```python
from build123d import *

# Parameters (mm, degrees)
SKETCH1_W           = 120
SKETCH1_H           = 70
BOSS_EXTRUDE1_DEPTH = 2
SKETCH3_R           = 3.5
CUT_EXTRUDE1_DEPTH  = 3
SKETCH6_R           = 2
BOSS_EXTRUDE2_DEPTH = 11
SKETCH4_R           = 3.25
CUT_EXTRUDE2_DEPTH  = 11


with BuildPart() as part:
    # Sketch1 → Boss-Extrude1 (new body)
    with BuildSketch(Plane(origin=(0, 0, 0), x_dir=(1, 0, 0), z_dir=(0, 1, 0))):
        Rectangle(SKETCH1_W, SKETCH1_H)
    extrude(amount=BOSS_EXTRUDE1_DEPTH)

    # Sketch3 → Cut-Extrude1 (cut)
    with BuildSketch(Plane(origin=(0, 2, 0), x_dir=(1, 0, 0), z_dir=(0, 1, 0))):
        with Locations(Location((-53.5, 28.5, 0), (0, 0, 270))):
            Circle(SKETCH3_R)
        with Locations(Location((53.5, 28.5, 0), (0, 0, 270))):
            Circle(SKETCH3_R)
        with Locations(Location((-53.5, -28.5, 0), (0, 0, 270))):
            Circle(SKETCH3_R)
        with Locations(Location((53.5, -28.5, 0), (0, 0, 270))):
            Circle(SKETCH3_R)
    extrude(amount=-CUT_EXTRUDE1_DEPTH, mode=Mode.SUBTRACT)

    # Sketch6 → Boss-Extrude2 (add)
    with BuildSketch(Plane(origin=(0, 2, 0), x_dir=(1, 0, 0), z_dir=(0, 1, 0))):
        with Locations(Location((0, -13, 0), (0, 0, 270))):
            Circle(SKETCH6_R)
        with Locations(Location((0, 13, 0), (0, 0, 270))):
            Circle(SKETCH6_R)
    extrude(amount=-BOSS_EXTRUDE2_DEPTH)

    # Sketch4 → Cut-Extrude2 (cut)
    with BuildSketch(Plane(origin=(0, 2, 0), x_dir=(1, 0, 0), z_dir=(0, 1, 0))):
        with Locations(Location((-27.054448087, -13.122273409, 0), (0, 0, 270))):
            Circle(SKETCH4_R)
        with Locations(Location((-27.023483048, -0.10764713, 0), (0, 0, 270))):
            Circle(SKETCH4_R)
        with Locations(Location((-27.081562274, 12.864019897, 0), (0, 0, 270))):
            Circle(SKETCH4_R)
        with Locations(Location((-13.567081484, 0, 0), (0, 0, 270))):
            Circle(SKETCH4_R)
        with Locations(Location((-13.567081484, -13, 0), (0, 0, 270))):
            Circle(SKETCH4_R)
        with Locations(Location((-13.567081484, 13, 0), (0, 0, 270))):
            Circle(SKETCH4_R)
        with Locations(Location((0, 0, 0), (0, 0, 270))):
            Circle(SKETCH4_R)
    extrude(amount=-CUT_EXTRUDE2_DEPTH, mode=Mode.SUBTRACT)


solid = part.part
```
Geometry: final body of the model. Coordinates: model frame, mm. A direction names the side the tool comes from. Coordinates: 2 decimals unless noted, no trailing zeros. Order: outer loops, then holes, each group sorted by start corner. A loop starts at its lowest first (then second) coordinate and runs counter-clockwise, first axis right, second up. Notation, with made-up numbers: (40.5, -36.75) - (66.5, -36.75) arc R23 cw to (66.5, -18.75) - close; hole circle Ø10 at (17.25, 3.25). An arc over 180 degrees is marked (long way). Return JSON: item names as keys, results as strings. Group by question number.
1. Cut plane A-A (z = 30). Output: boundary loops of the cut face in (x, y).
2. Cut plane B-B (x = 53.5). Output: boundary loops of the cut face in (y, z).
3. Material intervals for line 1 along X through (y, z) = (1.3, 13); line 2 along Y through (x, z) = (23, 2); line 3 along X through (y, z) = (-1.25, 13), sorted ascending. Write a range as [from, to].
4. Cut plane D-D (z = 0). Output: boundary loops of the cut face in (x, y), plus the area to 3 significant figures.
5. Set-up query: faces 1 (the face through (0, -9, -13)), 2 (the face through (-1.2, -4.4, -14.6)). Return all of +Z, -Z, +X, -X, +Y, -Y with unobstructed straight access to the full face (end or side cutting, diameter ignored); none if empty.
6. Pull-direction query (Z, two-part tool) for faces 3 (the face through (-50.55, 1.01, -26.62)), 4 (the face through (0, -9, 13)); classes: pulls with the +Z half, pulls with the -Z half, needs draft (parallel to the pull), parting line crosses it, or undercut.
7. Pin query (flat end, axial travel): pin 1 (8.5 mm diameter, centred on x = -13.57, z = 13, fed in from -Y); pin 2 (7.5 mm diameter, centred on x = -13.57, z = -13, fed in from +Y). Return the tip coordinate at first contact, or that it passes through.
8. Cut plane C-C (y = -7.75). Output: boundary loops of the cut face in (x, z), plus the area to 3 significant figures.
Resolved:
{
 "1": {"outline": "(-60, 0) - (-56.66, 0) - (-56.66, 2) - (-60, 2) - close; (-50.34, 0) - (50.34, 0) - (50.34, 2) - (-50.34, 2) - close; (56.66, 0) - (60, 0) - (60, 2) - (56.66, 2) - close"},
 "2": {"outline": "(0, -35) - (2, -35) - (2, -32) - (0, -32) - close; (0, -25) - (2, -25) - (2, 25) - (0, 25) - close; (0, 32) - (2, 32) - (2, 35) - (0, 35) - close"},
 "3": {"line 1": "x = [-60, -30.3], [-23.81, -16.82], [-10.32, 60]", "line 2": "y = [0, 2]", "line 3": "x = [-2, 2]"},
 "4": {"outline": "(-60, 0) - (-30.27, 0) - (-30.27, 2) - (-60, 2) - close; (-23.78, 0) - (-16.82, 0) - (-16.82, 2) - (-23.78, 2) - close; (-10.32, 0) - (-3.25, 0) - (-3.25, 2) - (-10.32, 2) - close; (3.25, 0) - (60, 0) - (60, 2) - (3.25, 2) - close", "area": "201 mm²"},
 "5": {"face 1": "+Z, -Z, +X, -X, -Y", "face 2": "-Y"},
 "6": {"face 3": "undercut", "face 4": "needs draft"},
 "7": {"pin 1": "stops at y = 0", "pin 2": "stops at y = 2"},
 "8": {"outline": "circle Ø4 at (0, -13); circle Ø4 at (0, 13)", "area": "25.1 mm²"}
}
